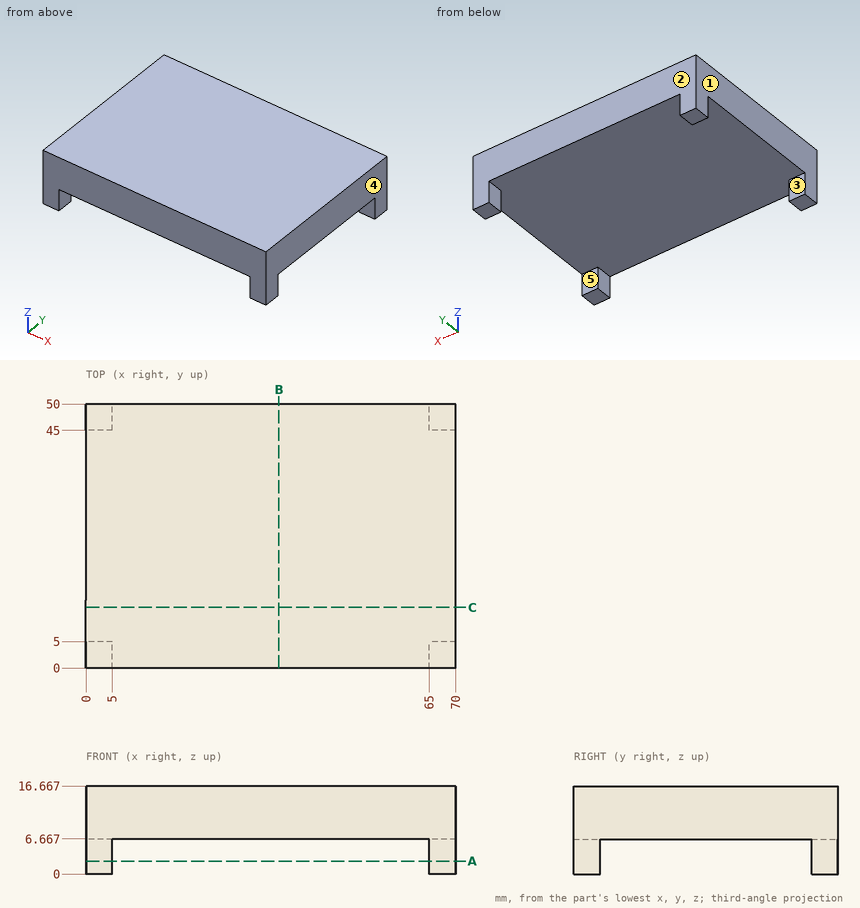
Geometry: see drawing. Coordinates: mm, zero at the bounding-box minimum. A direction names the side the tool comes from. Round coordinates to 2 decimals unless told otherwise and drop trailing zeros. Loops run counter-clockwise (first coordinate to the right, second up) from the corner with the lowest first, then second, coordinate; pieces in that order, holes last. Notation, with made-up numbers: (62, 69.5) -> (111, 69.5) arc R23 ccw to (111, 100.5) -> close; hole circle Ø8 at (37, 12). An arc over 180 degrees is marked (long way). One line per question, with ' | ' between items. Start each with the question number.
1. Mould query, pull axis Y, two halves, no side actions, for the marked faces 1, 2 and 3. Classes: pulls with the +Y half, pulls with the -Y half, needs draft (parallel to the pull), parting line crosses it, or undercut.
2. Section C-C on y = 11.5. Output: boundary loops of the cut face in (x, z).
3. Section B-B on x = 36.5. Output: boundary loops of the cut face in (y, z), and give its area (3 significant figures).
4. Set-up query: the marked faces 4 and 5. Return all of +Z, -Z, +X, -X, +Y, -Y with unobstructed straight access to the full face (end or side cutting, diameter ignored); none if empty.
5. Section A-A on z = 2.5. Output: boundary loops of the cut face in (x, y).
6. Contact query for a flat-ended pin moving along its axis: pin 1 (4 mm diameter, centred on x = 46.5, y = 10.5, fed in from -Z). Output: stop coordinate, or through.
7. Line query: line 1 along Z through (x, y) = (53, 21). Output: solid intervals per line, ascending. Write a range as [from, to].
Returned:
1) face 1: needs draft | face 2: pulls with the +Y half | face 3: undercut
2) outline: (0, 6.67) -> (70, 6.67) -> (70, 16.67) -> (0, 16.67) -> close
3) outline: (0, 6.67) -> (50, 6.67) -> (50, 16.67) -> (0, 16.67) -> close | area: 500 mm2
4) face 4: +Z, -Z, +X, +Y, -Y | face 5: -Z, +X, -X
5) outline: (0, 0) -> (5, 0) -> (5, 5) -> (0, 5) -> close; (0, 45) -> (5, 45) -> (5, 50) -> (0, 50) -> close; (65, 0) -> (70, 0) -> (70, 5) -> (65, 5) -> close; (65, 45) -> (70, 45) -> (70, 50) -> (65, 50) -> close
6) pin 1: stops at z = 6.67
7) line 1: z = [6.67, 16.67]
